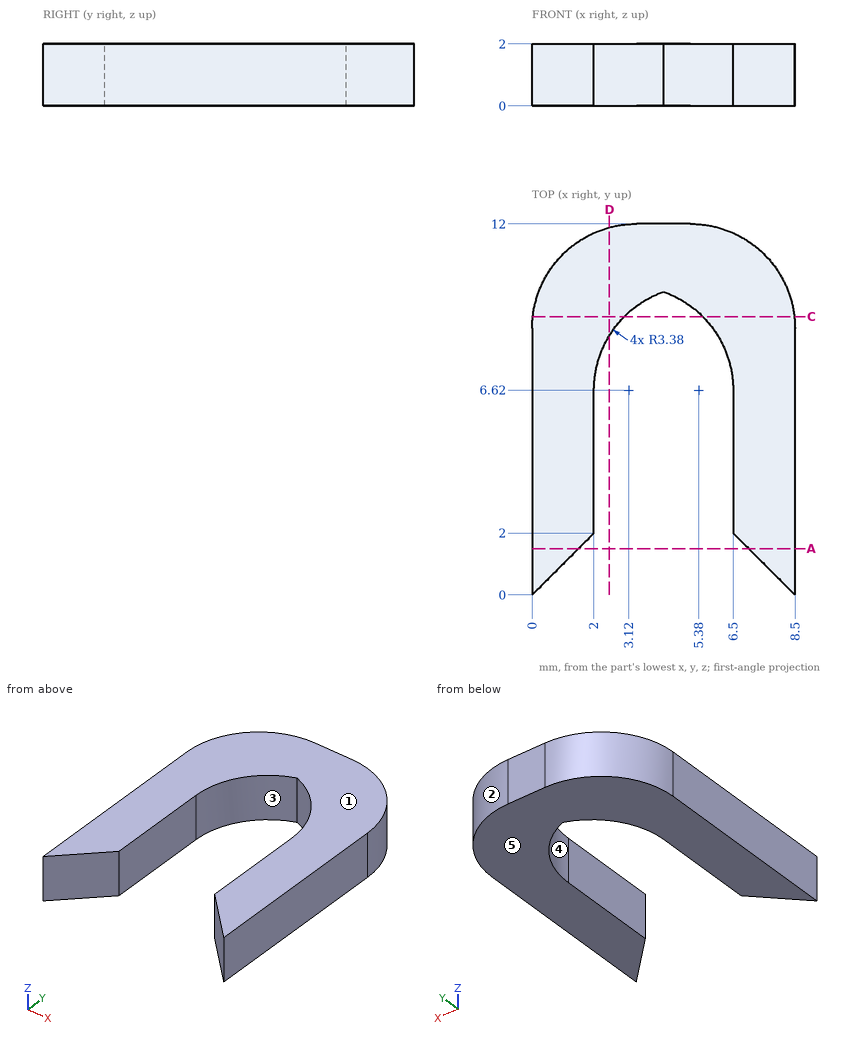
Source: three-view drawing plus pictorial views. Frame: mm from the lowest corner of the part. A direction names the side the tool comes from. Coordinates: 2 decimals unless noted, no trailing zeros. Loops run counter-clockwise (first coordinate to the right, second up) from the corner with the lowest first, then second, coordinate; pieces in that order, holes last. Notation, with made-up numbers: M -23,-19 L 14,-19 A10 ccw 14,-12 Z; hole C 77.25,64.5 d8. An arc over 180 degrees is marked long. Use CSV: the item, a comma, the result in double quotes.
(1) Line query: line 1 (X direction, y = 6.5, z = 1.3); line 2 (X direction, y = 9.5, z = 0.15); line 3 (Y direction, x = 4.5, z = 0.35). Output: solid intervals per line, ascending. Write a range as [from, to].
Answers follow:
line 1,"[0, 2], [6.5, 8.5]"
line 2,"[0.12, 3.61], [4.89, 8.38]"
line 3,"[9.71, 12]"
(2) Cut plane C-C on y = 9. Return loops of the section in (x, z), and give its area (3 significant figures).
Answers follow:
outline,"M 0.02,0 L 2.98,0 L 2.98,2 L 0.02,2 Z; M 5.52,0 L 8.48,0 L 8.48,2 L 5.52,2 Z"
area,"11.8 mm²"
(3) Cut plane D-D on x = 2.5. Return loops of the section in (y, z), and give its area (3 significant figures).
Answers follow:
outline,"M 8.39,0 L 11.88,0 L 11.88,2 L 8.39,2 Z"
area,"6.99 mm²"
(4) Cut plane A-A on y = 1.5. Return loops of the section in (x, z), and give its area (3 significant figures).
Answers follow:
outline,"M 0,0 L 1.5,0 L 1.5,2 L 0,2 Z; M 7,0 L 8.5,0 L 8.5,2 L 7,2 Z"
area,"6.00 mm²"
(5) Reachability of the marked faces 4 and 5 from +Z, -Z, +X, -X, +Y, -Y: full face, straight path, thin tool, end or side. Return the list, or none.
Answers follow:
face 4,"+Z, -Z, -Y"
face 5,"-Z, +X, -X, +Y, -Y"
(6) Draft query along X for the marked faces 1, 2 and 3. Return one class per face: pulls with the +X half, pulls with the -X half, needs draft (parallel to the pull), parting line crosses it, or undercut.
Answers follow:
face 1,"needs draft"
face 2,"pulls with the +X half"
face 3,"undercut"
